Here's how the part is built. I have some questions about the finished solid (model axes, mm). A direction names the side the tool comes from. Round coordinates to 2 decimals unless told otherwise and drop trailing zeros. Loops run counter-clockwise (first coordinate to the right, second up) from the corner with the lowest first, then second, coordinate; pieces in that order, holes last. Notation, with made-up numbers: M 44,44 L 71,44 A19 ccw 71,67 Z; hole C -13,48.25 d1. An arc over 180 degrees is marked long. Put each result on its own line as item: value. Start each with the question number.
Autodesk Inventor part; units mm, degrees
ref_plane "YZ Plane" through (0, 0, 0) normal (1, 0, 0) x (0, 1, 0)
ref_plane "XZ Plane" through (0, 0, 0) normal (0, 1, 0) x (-1, 0, 0)
ref_plane "XY Plane" through (0, 0, 0) normal (0, 0, 1) x (1, 0, 0)
sketch "Sketch1" plane through (0, 0, 0) normal (1, 0, 0) x (0, 1, 0)
  line L0 (-56, 56) -> (56, 56)
  line L1 (56, 56) -> (56, -56)
  line L2 (56, -56) -> (-56, -56)
  line L3 (-56, -56) -> (-56, 56)
  line L4 (-56, 56) -> (56, -56) construction
  line L5 (56, 56) -> (-56, -56) construction
  line L6 (-80, 80) -> (80, 80)
  line L7 (80, 80) -> (80, -80)
  line L8 (80, -80) -> (-80, -80)
  line L9 (-80, -80) -> (-80, 80)
  line L10 (-80, 80) -> (80, -80) construction
  line L11 (80, 80) -> (-80, -80) construction
  point P0 (0, 0)
  dimension "d0" = 112
  dimension "d1" = 112
  dimension "d2" = 160
  dimension "d3" = 160
extrude "Extrusion1" add sketch "Sketch1" along normal blind 35
extrude "Extrusion2" add sketch "Sketch1" against normal blind 5 contours L0 L1 L2 L3 | L6 L7 L8 L9
sketch "Sketch2" plane through (0, 0, 0) normal (1, 0, 0) x (0, 0, -1)
  circle A0 centre (0, 0) radius 45
  dimension "d8" = 90
extrude "Extrusion3" cut sketch "Sketch2" against normal through all
sketch "Sketch3" plane through (35, -80, 80) normal (0, 0, 1) x (1, 0, 0)
  line L0 (-35, 136) -> (-35, 24)
  line L1 (-35, 24) -> (0, 24)
  line L2 (-35, 136) -> (0, 136)
  line L3 (0, 0) -> (-40, 0)
  line L4 (-30, 0) -> (-30, 10)
  line L5 (-30, 10) -> (-10, 10)
  line L6 (-10, 10) -> (-10, 0)
  line L7 (0, 160) -> (0, 0)
  line L8 (-40, 0) -> (0, 0)
  line L9 (0, 160) -> (0, 0)
  line L10 (0, 160) -> (-40, 160)
  line L11 (-40, 0) -> (-40, 160)
  line L12 (-17.5, 80) -> (-40, 80)
  line L13 (-30, 0) -> (-10, 0)
  line L14 (-30, 160) -> (-30, 150)
  line L15 (-30, 150) -> (-10, 150)
  line L16 (-10, 150) -> (-10, 160)
  line L17 (-30, 160) -> (-10, 160)
  point P0 (-35, 80)
  dimension "d11" = 20
  dimension "d12" = 10
  dimension "d13" = 10
extrude "Extrusion4" cut sketch "Sketch3" against normal through all contours L16 L15 L14 L10 | L4 L5 L6 L3
sketch "Sketch4" plane through (35, -80, -80) normal (0, 0, -1) x (-1, 0, 0)
  line L0 (0, 0) -> (0, 160)
  line L1 (40, 160) -> (40, 0)
  line L2 (0, 0) -> (40, 0)
  line L3 (40, 0) -> (40, 160)
  line L4 (40, 160) -> (0, 160)
  line L5 (0, 160) -> (0, 0)
  point P0 (35, 80)
extrude "Extrusion5" cut sketch "Sketch4" against normal blind 20
sketch "Sketch5" plane through (25, -80, 80) normal (0, -1, 0) x (1, 0, 0)
  line L0 (-30, -140) -> (-30, 0)
  line L1 (-30, 0) -> (10, 0)
  line L2 (10, 0) -> (10, -140)
  line L3 (10, -140) -> (-30, -140)
  line L4 (-30, -140) -> (-30, 0)
  point P0 (-25, -80)
extrude "Extrusion6" cut sketch "Sketch5" against normal blind 10
sketch "Sketch6" plane through (25, 80, 80) normal (0, 1, 0) x (1, 0, 0)
  line L0 (10, 0) -> (0, 0)
  line L1 (-30, 0) -> (-30, 140)
  line L2 (10, 0) -> (-30, 0)
  line L3 (-30, 0) -> (-30, 140)
  line L4 (-30, 140) -> (10, 140)
  line L5 (10, 140) -> (10, 0)
  point P0 (-25, 80)
extrude "Extrusion7" cut sketch "Sketch6" against normal blind 10
sketch "Sketch7" plane through (-5, -70, 80) normal (0, -1, 0) x (1, 0, 0)
  line L0 (40, 0) -> (0, 0)
  line L1 (40, -140) -> (0, -140)
  line L2 (10, 0) -> (30, 0)
  line L3 (30, 0) -> (30, -140)
  line L4 (30, -140) -> (10, -140)
  line L5 (10, -140) -> (10, 0)
  point P0 (5, -80)
  dimension "d22" = 20
extrude "Extrusion8" cut sketch "Sketch7" against normal blind 4
sketch "Sketch8" plane through (-5, 70, 80) normal (0, 1, 0) x (1, 0, 0)
  line L0 (30, 0) -> (40, 0)
  line L1 (10, 140) -> (10, 0)
  line L2 (30, 0) -> (10, 0)
  line L3 (10, 0) -> (10, 140)
  line L4 (10, 140) -> (30, 140)
  line L5 (30, 140) -> (30, 0)
  point P0 (5, 80)
extrude "Extrusion9" cut sketch "Sketch8" against normal blind 4
properties part number "LeadScrewBox"
1) I'm going to push flat-ended pins straight in: P1, Ø2, axis at x = 23, z = -22, coming from the +Y side; P2, Ø10, axis at x = 12.5, z = -3, coming from the -Y side. Where does each tip first touch, or does it pass through?
2) If I drill on probe 1 along Y at (x, z) = (-1.95, 0); probe 2 along Z at (x, y) = (22, 38); probe 3 along Y at (x, z) = (24.5, 34), over which ranges is the centre line in solid material (lowest first)? Write a range as from..to.
3) On a 3-axis mill with a long thin cutter (end or side, diameter ignored), from which of +Z, -Z, +X, -X, +Y, -Y can I reach the whole of each face in a straight line? I mean faces 1 (the face through (5, 68, 9)), 2 (the face through (17, 56, 1)), 3 (the face through (25, -68, 11)). Say none if no direction works.
4) Suppose I cut it at A-A (x = 29). Write out the boundary of the cut face in (y, z).
5) Suppose I cut it at B-B (y = 0). Write out the boundary of the cut face in (x, z), plus the area to 3 significant figures.
6) If we mould it in two halves opening along X, with no side actions, what happens to faces 4 (the face through (0, -26, 38)), 5 (the face through (17, 1, -56)), 6 (the face through (15, 66, 9))? For each: pulls with the +X half, pulls with the -X half, needs draft (parallel to the pull), parting line crosses it, or undercut.
7) Suppose I cut it at C-C (z = 0). Write out the boundary of the cut face in (x, y), plus the area to 3 significant figures.
8) Suppose I cut it at D-D (y = 26.5). Write out the boundary of the cut face in (x, z).
Results are:
1. P1: y = 66
1. P2: y = -66
2. probe 1: -70..-45, 45..70
2. probe 2: -60..-56, 56..80
2. probe 3: -66..-56, 56..66
3. face 1: +Z, -Z, +Y
3. face 2: +X
3. face 3: +Z, -Z, -Y
4. outline: M -70,-60 L 70,-60 L 70,80 L -70,80 Z; hole M -56,-56 L 56,-56 L 56,56 L -56,56 Z
5. outline: M -5,-60 L 35,-60 L 35,-56 L 0,-56 L 0,-45 L -5,-45 Z; M -5,45 L 0,45 L 0,56 L 35,56 L 35,80 L -5,80 Z
5. area: 1,230 mm²
6. face 4: pulls with the +X half
6. face 5: needs draft
6. face 6: undercut
7. outline: M -5,-70 L 5,-70 L 5,-66 L 25,-66 L 25,-70 L 35,-70 L 35,-56 L 0,-56 L 0,-45 L -5,-45 Z; M -5,45 L 0,45 L 0,56 L 35,56 L 35,70 L 25,70 L 25,66 L 5,66 L 5,70 L -5,70 Z
7. area: 1,070 mm²
8. outline: M -5,-60 L 35,-60 L 35,-56 L 0,-56 L 0,-36.37 L -5,-36.37 Z; M -5,36.37 L 0,36.37 L 0,56 L 35,56 L 35,80 L -5,80 Z
